from build123d import *

# Parameters (mm, degrees)
SKETCH1_R             = 3.175
BOSS_EXTRUDE1_DEPTH   = 31.75
BOSS_EXTRUDE1_2_DEPTH = 31.75
BOSS_EXTRUDE2_START   = 20
BOSS_EXTRUDE2_DEPTH   = 20
CUT_EXTRUDE2_DEPTH    = 46.173478115
SKETCH4_R             = 2
CUT_EXTRUDE3_DEPTH    = 3.175


with BuildPart() as part:
    # Sketch1 → Boss-Extrude1 (new body)
    with BuildSketch(Plane(origin=(0, 0, 0), x_dir=(1, 0, 0), z_dir=(0, 1, 0))):
        with Locations(Location((-15, 0, 0), (0, 0, 270))):
            Circle(SKETCH1_R)
    extrude(amount=BOSS_EXTRUDE1_DEPTH)



with BuildPart() as body_2:
    # Sketch1 → Boss-Extrude1 2 (new body)
    with BuildSketch(Plane(origin=(0, 0, 0), x_dir=(1, 0, 0), z_dir=(0, 1, 0))):
        with Locations(Location((15, 0, 0), (0, 0, 270))):
            Circle(SKETCH1_R)
    extrude(amount=BOSS_EXTRUDE1_2_DEPTH)


with BuildPart() as part_1:
    add(part.part)

    add(body_2.part)  # Boss-Extrude2 merges body 2
    # Sketch2 → Boss-Extrude2 (add)
    with BuildSketch(Plane.XZ.offset(BOSS_EXTRUDE2_START)):
        with BuildLine():
            Line((-15, 3.175), (-15, 13.25))
            Line((-15, 13.25), (15, 13.25))
            Line((15, 13.25), (15, 3.175))
            ThreePointArc((15, 3.175), (18.175, 0), (15, -3.175))
            Line((15, -3.175), (15, -13.25))
            Line((15, -13.25), (-15, -13.25))
            Line((-15, -13.25), (-15, -3.175))
            ThreePointArc((-15, -3.175), (-18.175, 0), (-15, 3.175))
        make_face()
    extrude(amount=-BOSS_EXTRUDE2_DEPTH)

    # Sketch5 → Cut-Extrude2 (cut, through all)
    with BuildSketch(Plane.XY.offset(13.25)):
        with BuildLine():
            ThreePointArc((15, -4.692512186), (0, -11.35), (-15, -4.692512186))
            Line((-15, -4.692512186), (-15, -20))
            Line((-15, -20), (15, -20))
            Line((15, -20), (15, -4.692512186))
        make_face()
        with BuildLine():
            ThreePointArc((-15, -4.692512186), (-16.752613942, -2.457973814), (-18.175, 0))
            Line((-18.175, 0), (-18.175, -20))
            Line((-18.175, -20), (-15, -20))
            Line((-15, -20), (-15, -4.692512186))
        make_face()
        with BuildLine():
            ThreePointArc((18.175, 0), (16.752613942, -2.457973814), (15, -4.692512186))
            Line((15, -4.692512186), (15, -20))
            Line((15, -20), (18.175, -20))
            Line((18.175, -20), (18.175, 0))
        make_face()
        with BuildLine():
            ThreePointArc((-11.825, 0), (0, -5), (11.825, 0))
            Line((11.825, 0), (-11.825, 0))
        make_face()
    extrude(amount=-CUT_EXTRUDE2_DEPTH, mode=Mode.SUBTRACT)

    # Sketch4 → Cut-Extrude3 (cut)
    with BuildSketch(Plane(origin=(0, 31.75, 0), x_dir=(1, 0, 0), z_dir=(0, 1, 0))):
        with Locations(Location((-15, 0, 0), (0, 0, 270))):
            Circle(SKETCH4_R)
        with Locations(Location((15, 0, 0), (0, 0, 270))):
            Circle(SKETCH4_R)
    extrude(amount=-CUT_EXTRUDE3_DEPTH, mode=Mode.SUBTRACT)


solid = part_1.part
Verification items for the finished model (mm, model axes). A direction names the side the tool comes from. Coordinates: 2 decimals unless noted, no trailing zeros. Order: outer loops, then holes, each group sorted by start corner. A loop starts at its lowest first (then second) coordinate and runs counter-clockwise, first axis right, second up.
1. Sectioned sample at D-D, the plane x = -12.5. Record the cut outline in (y, z).
Results found:
outline: (-7.03, -13.25) - (0, -13.25) - (0, -1.96) - (31.75, -1.96) - (31.75, 1.96) - (0, 1.96) - (0, 13.25) - (-7.03, 13.25) - close
2. Release check for a two-part mould opening along X. For faces 1 (the face through (15, -2, 8)), 2 (the face through (18.15, 13.27, -0.41)), 3 (the face through (-15, -2, 8)) record: +X half, -X half, draft (parallel to the pull), parting line (faces both ways), or undercut.
Results found:
face 1: +X half
face 2: undercut
face 3: -X half
3. Go/stop test with flat-tipped pins: pin 1 Ø4 at (y, z) = (24, 2.5) entering from +X; pin 2 Ø4 at (y, z) = (0.5, -9.5) entering from +X; pin 3 Ø2 at (x, z) = (15.5, -0.5) entering from +Y (3 decimals). Record where each tip stops, or that it passes through.
Results found:
pin 1: stops at x = 18.14
pin 2: stops at x = 15
pin 3: stops at y = 28.575
4. Sectioned sample at A-A, the plane y = 9.5. Record the cut outline in (x, z) (3 decimals), and give its area (3 significant figures).
Results found:
outline: circle Ø6.35 at (-15, 0); circle Ø6.35 at (15, 0)
area: 63.3 mm2
5. Sectioned sample at C-C, the plane x = 14. Record the cut outline in (y, z) (3 decimals), and give its area (3 significant figures).
Results found:
outline: (-5.722, -13.25) - (0, -13.25) - (0, -3.013) - (31.75, -3.013) - (31.75, -1.732) - (28.575, -1.732) - (28.575, 1.732) - (31.75, 1.732) - (31.75, 3.013) - (0, 3.013) - (0, 13.25) - (-5.722, 13.25) - close
area: 332 mm2
6. Sectioned sample at B-B, the plane z = -8.5. Record the cut outline in (x, y) (3 decimals).
Results found:
outline: (-15, -4.693) arc R20.227 ccw to (15, -4.693) - (15, 0) - (11.825, 0) arc R16.483 cw to (-11.825, 0) - (-15, 0) - close
7. Scan lines: line 1 (X direction, y = 30.1, z = 0) (3 decimals); line 2 (Z direction, x = 15, y = 12.5) (3 decimals); line 3 (Y direction, x = -0.5, z = -3.75). Record each from-to range of solid material in increasing order.
Results found:
line 1: x = -18.175 to -17, -13 to -11.825, 11.825 to 13, 17 to 18.175
line 2: z = -3.175 to 3.175
line 3: y = -11.34 to -4.99
8. Set-up check for faces 4 (the face through (15, 28.575, 0)), 5 (the face through (15, -2, -8)), 6 (the face through (-15, -2, -8)): record each of +Z, -Z, +X, -X, +Y, -Y from which the full face is reachable in a straight line by a thin tool's end or side.
Results found:
face 4: +Y
face 5: -Z, +X, +Y, -Y
face 6: -Z, -X, +Y, -Y
